Work out the finished part from the listing and answer in its coordinate system (mm). Round coordinates to 2 decimals unless told otherwise and drop trailing zeros. Loops run counter-clockwise (first coordinate to the right, second up) from the corner with the lowest first, then second, coordinate; pieces in that order, holes last.
```python
from build123d import *

# Parameters (mm, degrees)
F0_W     = 50.8
F0_H     = 177.8
F1_DEPTH = 9.525
F2_D     = 5.1054
F3_D     = 10.0838


# Not quite as in the source:
# - a length typed as a fraction of an inch, garbled in the dataset ("3 / 203.2 mm" for 3/8 in), is restored


with BuildPart() as f1:
    # F0 (on Top) → F1 (new body)
    with BuildSketch(Plane.XY):
        with Locations((-25.4, 88.9)):
            Rectangle(F0_W, F0_H)
    extrude(amount=-F1_DEPTH)

    # F2 (through all)
    with Locations(Plane.XY):
        with Locations((-12.7, 12.7), (-25.4, 12.7), (-38.1, 12.7), (-38.1, 25.4), (-25.4, 25.4), (-12.7, 25.4), (-12.7, 38.1), (-25.4, 38.1), (-38.1, 38.1), (-38.1, 50.8), (-25.4, 50.8), (-12.7, 50.8)):
            Hole(F2_D / 2)

    # F3 (through all)
    with Locations(Plane.XY):
        with Locations((-38.1, 161.925)):
            Hole(F3_D / 2)


solid = f1.part
```
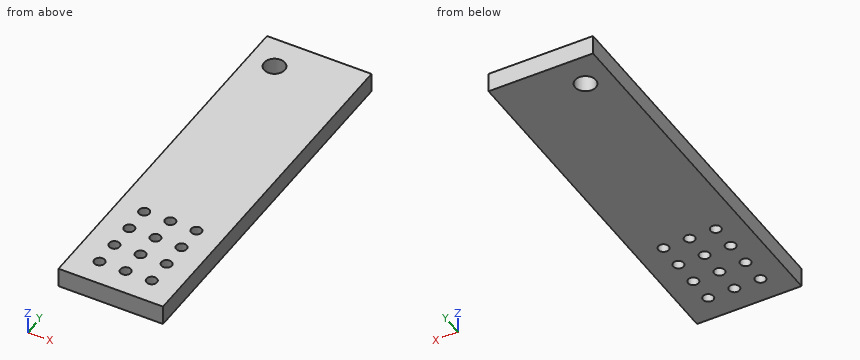
1. Find section D-D (z = -5.25). Give the number of separate pieces and of enclosed holes in the cut face, then the cut area to 3 significant figures.
Answer key:
separate pieces: 1
enclosed holes: 13
area: 8,710 mm2
2. Find section A-A (y = 25.4). Write down the section's boundary in (x, z) (3 decimals), then the cut area to 3 significant figures.
Answer key:
outline: (-50.8, -9.525) - (-40.653, -9.525) - (-40.653, 0) - (-50.8, 0) - close; (-35.547, -9.525) - (-27.953, -9.525) - (-27.953, 0) - (-35.547, 0) - close; (-22.847, -9.525) - (-15.253, -9.525) - (-15.253, 0) - (-22.847, 0) - close; (-10.147, -9.525) - (0, -9.525) - (0, 0) - (-10.147, 0) - close
area: 338 mm2
3. Find section B-B (x = -25.4). Write down the section's boundary in (y, z) (3 decimals).
Answer key:
outline: (0, -9.525) - (10.147, -9.525) - (10.147, 0) - (0, 0) - close; (15.253, -9.525) - (22.847, -9.525) - (22.847, 0) - (15.253, 0) - close; (27.953, -9.525) - (35.547, -9.525) - (35.547, 0) - (27.953, 0) - close; (40.653, -9.525) - (48.247, -9.525) - (48.247, 0) - (40.653, 0) - close; (53.353, -9.525) - (177.8, -9.525) - (177.8, 0) - (53.353, 0) - close
4. Find section C-C (x = -38.1). Write down the section's boundary in (y, z) (3 decimals), then the cut area to 3 significant figures.
Answer key:
outline: (0, -9.525) - (10.147, -9.525) - (10.147, 0) - (0, 0) - close; (15.253, -9.525) - (22.847, -9.525) - (22.847, 0) - (15.253, 0) - close; (27.953, -9.525) - (35.547, -9.525) - (35.547, 0) - (27.953, 0) - close; (40.653, -9.525) - (48.247, -9.525) - (48.247, 0) - (40.653, 0) - close; (53.353, -9.525) - (156.883, -9.525) - (156.883, 0) - (53.353, 0) - close; (166.967, -9.525) - (177.8, -9.525) - (177.8, 0) - (166.967, 0) - close
area: 1,400 mm2
5. Consider probe 1 along Y at (x, z) = (-25, -2); probe 2 along Y at (x, z) = (-38, -1.5); probe 3 along Y at (x, z) = (-27.5, -4). Determine where each line is inside the solid, lowest interval first.
Answer key:
probe 1: y = 0 to 10.18, 15.22 to 22.88, 27.92 to 35.58, 40.62 to 48.28, 53.32 to 177.8
probe 2: y = 0 to 10.15, 15.25 to 22.85, 27.95 to 35.55, 40.65 to 48.25, 53.35 to 156.88, 166.97 to 177.8
probe 3: y = 0 to 11.25, 14.15 to 23.95, 26.85 to 36.65, 39.55 to 49.35, 52.25 to 177.8
6. Given pin 1 (3 mm diameter, centred on x = -25.4, y = 12.7, fed in from +Z); pin 2 (1 mm diameter, centred on y = 90.5, z = -7.5, fed in from +X), each flat-ended and moving along its own axis, determine where each tip first touches the part or whether it passes through.
Answer key:
pin 1: passes through
pin 2: stops at x = 0
